```python
from build123d import *

# Parameters (mm, degrees)
SKETCH1_R                      = 12
BOSS_EXTRUDE1_DEPTH            = 3
BOSS_EXTRUDE2_START            = 37
SKETCH1_3_W                    = 115.5
SKETCH1_3_H                    = 30.5
BOSS_EXTRUDE2_DEPTH            = 37
BOSS_EXTRUDE3_DEPTH            = 33.5
BOSS_EXTRUDE3_DEPTH_BACK       = 3
CBORE_FOR_M5_SHCS1_D           = 5.3
CBORE_FOR_M5_SHCS1_CBORE_D     = 10
CBORE_FOR_M5_SHCS1_CBORE_DEPTH = 9.75
FILLET1_R                      = 2
FILLET2_R                      = 1.5


with BuildPart() as part:
    # Sketch1 → Boss-Extrude1 (new body)
    with BuildSketch(Plane.XY):
        with BuildLine():
            Line((-3, -3), (118.5, -3))
            Line((118.5, -3), (118.5, 33.5))
            Line((118.5, 33.5), (0, 33.5))
            ThreePointArc((0, 33.5), (-0.773900275, 33.398461379), (-1.495413373, 33.100718909))
            Line((-1.495413373, 33.100718909), (-21.495413373, 21.600718909))
            ThreePointArc((-21.495413373, 21.600718909), (-22.596751829, 20.502291563), (-23, 19))
            Line((-23, 19), (-23, 17))
            Line((-23, 17), (-3, 17))
            Line((-3, 17), (-3, 9.4))
            Line((-3, 9.4), (-5, 9.4))
            Line((-5, 9.4), (-5, 4.6))
            Line((-5, 4.6), (-3, 4.6))
            Line((-3, 4.6), (-3, -3))
        make_face()
        with Locations((57.75, 15.25)):
            Circle(SKETCH1_R, mode=Mode.SUBTRACT)
        with Locations((22.75, 15.25)):
            Circle(SKETCH1_R, mode=Mode.SUBTRACT)
        with Locations((92.75, 15.25)):
            Circle(SKETCH1_R, mode=Mode.SUBTRACT)
    extrude(amount=-BOSS_EXTRUDE1_DEPTH)

    # Sketch1<3> → Boss-Extrude2 (add)
    with BuildSketch(Plane.XY.offset(BOSS_EXTRUDE2_START)):
        with BuildLine():
            Line((-3, -3), (118.5, -3))
            Line((118.5, -3), (118.5, 33.5))
            Line((118.5, 33.5), (0, 33.5))
            ThreePointArc((0, 33.5), (-0.773900275, 33.398461379), (-1.495413373, 33.100718909))
            Line((-1.495413373, 33.100718909), (-21.495413373, 21.600718909))
            ThreePointArc((-21.495413373, 21.600718909), (-22.596751829, 20.502291563), (-23, 19))
            Line((-23, 19), (-23, 17))
            Line((-23, 17), (-3, 17))
            Line((-3, 17), (-3, 9.4))
            Line((-3, 9.4), (-5, 9.4))
            Line((-5, 9.4), (-5, 4.6))
            Line((-5, 4.6), (-3, 4.6))
            Line((-3, 4.6), (-3, -3))
        make_face()
        with Locations((57.75, 15.25)):
            Rectangle(SKETCH1_3_W, SKETCH1_3_H, mode=Mode.SUBTRACT)
    extrude(amount=-BOSS_EXTRUDE2_DEPTH)


with BuildPart() as body_2:
    # Sketch2 → Boss-Extrude3 (new, two sides: drawn at the far end of the back side and taken through both)
    with BuildSketch(Plane(origin=(0, 0, 0), x_dir=(1, 0, 0), z_dir=(0, 1, 0)).offset(-BOSS_EXTRUDE3_DEPTH_BACK)):
        with BuildLine():
            Line((-23, -37), (8.597499345, -37))
            ThreePointArc((8.597499345, -37), (19.597359516, -22.852490863), (36.699987142, -17.500008554))
            Line((36.699987142, -17.500008554), (118.5, -17.500008554))
            Line((118.5, -17.500008554), (118.5, 3))
            Line((118.5, 3), (-23, 3))
            Line((-23, 3), (-23, -37))
        make_face()
    extrude(amount=BOSS_EXTRUDE3_DEPTH + BOSS_EXTRUDE3_DEPTH_BACK)


with BuildPart() as part_1:
    add(part.part)

    # Combine1: intersect body 2
    add(body_2.part, mode=Mode.INTERSECT)

    # CBORE for M5 SHCS1 (through all)
    with Locations(Plane(origin=(0, 33.5, 0), x_dir=(1, 0, 0), z_dir=(0, 1, 0))):
        with Locations((-13, -7), (-13, -27)):
            CounterBoreHole(CBORE_FOR_M5_SHCS1_D / 2, CBORE_FOR_M5_SHCS1_CBORE_D / 2, CBORE_FOR_M5_SHCS1_CBORE_DEPTH)

    # Fillet1
    fillet1_edges = [part_1.edges().sort_by_distance(p)[0] for p in [
        (8.597499345, -1.5, 37),
        (115.5, 0, 8.750004277),
        (8.597499345, 32, 37),
        (-23, 18, -3),
        (118.5, 33.5, 7.250004277),
        (118.5, -3, 7.250004277),
        (57.75, -3, -3),
        (118.5, 15.25, -3),
        (0, 0, 18.5),
        (59.25, 33.5, -3),
        (57.75, 0, 0),
        (-0.773900275, 33.398461379, -3),
        (-11.495413373, 27.350718909, -3),
        (-22.596751829, 20.502291563, -3),
    ]]
    fillet(fillet1_edges, radius=FILLET1_R)

    # Fillet2
    fillet2_edges = [part_1.edges().sort_by_distance(p)[0] for p in [
        (-3, 17, 17),
    ]]
    fillet(fillet2_edges, radius=FILLET2_R)


solid = part_1.part
```
The listing builds one solid part. Answer for the finished solid, in the listing's coordinates (mm). A direction names the side the tool comes from. Give positions to 0.01 mm unless a question says otherwise; leave off trailing zeros. Order: outer loops, then holes, each group sorted by start corner. A loop starts at its lowest first (then second) coordinate and runs counter-clockwise, first axis right, second up.
1) Find section B-B on x = 57.75. Write down the section's boundary in (y, z), then the cut area to 3 significant figures.
Reported:
outline: (-3, -1) arc R2 ccw to (-1, -3) - (3.25, -3) - (3.25, 0) - (2, 0) arc R2 cw to (0, 2) - (0, 17.5) - (-3, 17.5) - close; (27.25, -3) - (31.5, -3) arc R2 ccw to (33.5, -1) - (33.5, 17.5) - (30.5, 17.5) - (30.5, 0) - (27.25, 0) - close
area: 142 mm2
2) Find section A-A on z = 7. Give the number of separate pieces and of enclosed holes in the cut face, then the cut area to 3 significant figures.
Reported:
separate pieces: 2
enclosed holes: 1
area: 1,050 mm2
3) Consider line 1 along Z through (x, y) = (-13, 21.75); line 2 along Y through (x, z) = (67.5, 3); line 3 along Z through (x, y) = (37.5, 31.5). Determine where each line is inside the solid, lowest interval first.
Reported:
line 1: z = -3 to 4.35, 9.65 to 24.35, 29.65 to 37
line 2: y = -3 to 0, 30.5 to 33.5
line 3: z = -3 to 17.5
4) Find section D-D on y = 13. Write down the section's boundary in (x, z), then the cut area to 3 significant figures.
Reported:
outline: (-3, -3) - (10.96, -3) - (10.96, 0) - (0, 0) - (0, 37) - (-3, 37) - close; (34.54, -3) - (45.96, -3) - (45.96, 0) - (34.54, 0) - close; (69.54, -3) - (80.96, -3) - (80.96, 0) - (69.54, 0) - close; (104.54, -3) - (116.5, -3) arc R2 ccw to (118.5, -1) - (118.5, 17.5) - (115.5, 17.5) - (115.5, 0) - (104.54, 0) - close
area: 315 mm2
5) Determine the mould class of faces 6 (the face through (45, 0, 12)), 7 (the face through (19.94, 31.98, 22.62)), 8 (the face through (-5, 7, 17)) for opening direction X: pulls with the +X half, pulls with the -X half, needs draft (parallel to the pull), parting line crosses it, or undercut.
Reported:
face 6: undercut
face 7: pulls with the +X half
face 8: pulls with the -X half
6) For faces 1 (the face through (115.5, 16, 9)), 2 (the face through (-3, 1, 17)), 3 (the face through (-3, 12, 17)), 4 (the face through (-11.351, 26.776, -2.399)), 5 (the face through (-15, 23.75, 9)), determine the directions among +Z, -Z, +X, -X, +Y, -Y from which every point of the face is accessible in a straight line to the end or side of a thin tool.
Reported:
face 1: +Z
face 2: +Z, -Z, -X, -Y
face 3: +Z, -Z, -X
face 4: -Z, -X, +Y
face 5: +Y
7) Find section C-C on x = 42.5. Write down the section's boundary in (y, z).
Reported:
outline: (-3, -1) arc R2 ccw to (-1, -3) - (31.5, -3) arc R2 ccw to (33.5, -1) - (33.5, 17.5) - (30.5, 17.5) - (30.5, 0) - (2, 0) arc R2 cw to (0, 2) - (0, 17.5) - (-3, 17.5) - close
8) Given P1, Ø6, axis at x = -13, z = 7, coming from the -Y side; P2, Ø8, axis at x = -11.5, z = 26.5, coming from the +Y side; P3, Ø4, axis at y = 1, z = 7.5, coming from the -X side; P4, Ø4, axis at x = -13, z = 27, coming from the +Y side, each flat-ended and moving along its own axis, determine where each tip first touches the part or whether it passes through.
Reported:
P1: stops at y = 17
P2: stops at y = 29.65
P3: stops at x = -3
P4: passes through
